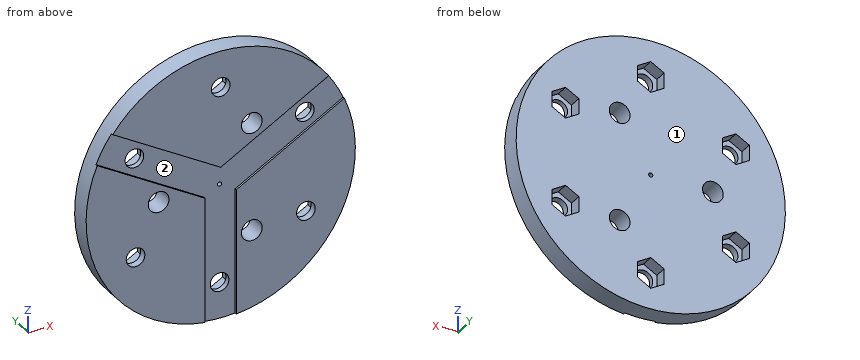
from build123d import *

# Parameters (mm, degrees)
SKETCH1_R           = 65
SKETCH1_R_2         = 1
BOSS_EXTRUDE1_DEPTH = 5
CUT_EXTRUDE1_DEPTH  = 6.4
SKETCH4_R           = 4.5
CUT_EXTRUDE2_DEPTH  = 93.146405247
CUT_EXTRUDE3_START  = -9
CUT_EXTRUDE3_DEPTH  = 3
SKETCH6_R           = 5
CUT_EXTRUDE4_DEPTH  = 93.466210045


with BuildPart() as part:
    # Sketch1 → Boss-Extrude1 (new, symmetric)
    with BuildSketch(Plane(origin=(0, 0, 0), x_dir=(1, 0, 0), z_dir=(0, 1, 0))):
        with Locations(Location((0, 0, 0), (0, 0, 270))):
            Circle(SKETCH1_R)
        with Locations(Location((0, 0, 0), (0, 0, 270))):
            Circle(SKETCH1_R_2, mode=Mode.SUBTRACT)
    extrude(amount=BOSS_EXTRUDE1_DEPTH, both=True)

    # Sketch3 → Cut-Extrude1 (cut)
    with BuildSketch(Plane(origin=(0, 5, 0), x_dir=(1, 0, 0), z_dir=(0, 1, 0))):
        Polygon((34.68620668, 20.026090764), (41.13620668, 16.302181527), (47.58620668, 20.026090764), (47.58620668, 27.473909236), (41.13620668, 31.197818473), (34.68620668, 27.473909236), align=None)
        Polygon((0, 40.052181527), (6.45, 43.776090764), (6.45, 51.223909236), (0, 54.947818473), (-6.45, 51.223909236), (-6.45, 43.776090764), align=None)
        Polygon((34.68620668, -20.026090764), (34.68620668, -27.473909236), (41.13620668, -31.197818473), (47.58620668, -27.473909236), (47.58620668, -20.026090764), (41.13620668, -16.302181527), align=None)
        Polygon((0, -40.052181527), (-6.45, -43.776090764), (-6.45, -51.223909236), (0, -54.947818473), (6.45, -51.223909236), (6.45, -43.776090764), align=None)
        Polygon((-34.68620668, -20.026090764), (-41.13620668, -16.302181527), (-47.58620668, -20.026090764), (-47.58620668, -27.473909236), (-41.13620668, -31.197818473), (-34.68620668, -27.473909236), align=None)
        Polygon((-34.68620668, 20.026090764), (-34.68620668, 27.473909236), (-41.13620668, 31.197818473), (-47.58620668, 27.473909236), (-47.58620668, 20.026090764), (-41.13620668, 16.302181527), align=None)
    extrude(amount=-CUT_EXTRUDE1_DEPTH, mode=Mode.SUBTRACT)

    # Sketch4 → Cut-Extrude2 (cut, through all)
    with BuildSketch(Plane(origin=(0, -1.4, 0), x_dir=(1, 0, 0), z_dir=(0, 1, 0))):
        with Locations(Location((0, 47.5, 0), (0, 0, 270))):
            Circle(SKETCH4_R)
        with Locations(Location((41.13620668, 23.75, 0), (0, 0, 270))):
            Circle(SKETCH4_R)
        with Locations(Location((41.13620668, -23.75, 0), (0, 0, 270))):
            Circle(SKETCH4_R)
        with Locations(Location((0, -47.5, 0), (0, 0, 270))):
            Circle(SKETCH4_R)
        with Locations(Location((-41.13620668, -23.75, 0), (0, 0, 270))):
            Circle(SKETCH4_R)
        with Locations(Location((-41.13620668, 23.75, 0), (0, 0, 270))):
            Circle(SKETCH4_R)
    extrude(amount=-CUT_EXTRUDE2_DEPTH, mode=Mode.SUBTRACT)

    # Sketch5 → Cut-Extrude3 (cut)
    with BuildSketch(Plane(origin=(0, 5, 0), x_dir=(1, 0, 0), z_dir=(0, 1, 0)).offset(CUT_EXTRUDE3_START)):
        Polygon((60.463542815, -26.248388682), (7.5, 4.330127019), (7.5, 65.487158421), (-7.5, 65.487158421), (-7.5, 4.330127019), (-60.463542815, -26.248388682), (-52.963542815, -39.238769739), (0, -8.660254038), (52.963542815, -39.238769739), align=None)
    extrude(amount=-CUT_EXTRUDE3_DEPTH, mode=Mode.SUBTRACT)

    # Sketch6 → Cut-Extrude4 (cut, through all)
    with BuildSketch(Plane.XZ.offset(5)):
        with Locations(Location((-30, 0, 0), (0, 0, 270))):
            Circle(SKETCH6_R)
        with Locations(Location((15, 25.980762114, 0), (0, 0, 270))):
            Circle(SKETCH6_R)
        with Locations(Location((15, -25.980762114, 0), (0, 0, 270))):
            Circle(SKETCH6_R)
    extrude(amount=-CUT_EXTRUDE4_DEPTH, mode=Mode.SUBTRACT)


solid = part.part
Model file for the job. Use its own axes, mm. Face numbers are marked on the shaded views. Coordinates: 2 decimals unless noted, no trailing zeros. Write each loop counter-clockwise with the first axis right and the second up, starting at its lowest first coordinate (ties: lowest second). Pieces come first, ordered by that corner, then holes. Notation, with made-up numbers: (-1.5, 35.25) -> (41.5, 35.25) arc R37 cw to (41.5, 71.25) -> close; hole circle Ø2 at (-0.5, 78). An arc over 180 degrees is marked (long way). One line per item, written item: value. Start each with the question number.
1) Probe probe 1 along X at (y, z) = (0.75, 0); probe 2 along Z at (x, y) = (3.5, 0.75); probe 3 along X at (y, z) = (3.25, -17). List the from-to ranges inside material, lowest first.
2) Slice it at C-C on x = -30. Write the cut outline in (y, z).
3) Flat gauge pins, fed straight in: pin 1 Ø2 at (x, y) = (-36, 4) entering from -Z; pin 2 Ø5 at (y, z) = (0.5, 24.5) entering from +X; pin 3 Ø5 at (x, y) = (-13, 1.5) entering from -Z. Where does each tip first touch, or does it go through?
4) Pull direction Z, two halves, no side cores. Call the marked faces 1 and 2: +Z half, -Z half, draft (parallel to the pull), parting line (faces both ways), or undercut.
5) Slice it at B-B on z = 23.75. Count the separate pieces of the cut face and the enclosed holes in it, then the cut area to 3 significant figures.
6) Slice it at A-A on x = 15. Write the cut outline in (y, z).
7) Slice it at D-D on z = -47.5. Write the cut outline in (x, y).
Answers follow:
1. probe 1: -65 to -35, -25 to -1, 1 to 65
1. probe 2: -64.91 to -52.93, -42.07 to 42.07, 52.93 to 64.91
1. probe 3: -62.74 to -42.34, -39.93 to 39.93, 42.34 to 62.74
2. outline: (-5, -57.66) -> (5, -57.66) -> (5, -5) -> (-5, -5) -> close; (-5, 5) -> (5, 5) -> (5, 57.66) -> (-5, 57.66) -> (-5, 25.98) -> (-4, 25.98) -> (-4, 8.66) -> (-5, 8.66) -> close
3. pin 1: z = -54.77
3. pin 2: x = 61.16
3. pin 3: z = -64.15
4. face 1: draft
4. face 2: undercut
5. separate pieces: 4
5. enclosed holes: 0
5. area: 849 mm2
6. outline: (-5, -63.25) -> (5, -63.25) -> (5, -30.98) -> (-5, -30.98) -> close; (-5, -20.98) -> (5, -20.98) -> (5, 20.98) -> (-5, 20.98) -> (-5, 17.32) -> (-4, 17.32) -> (-4, 0) -> (-5, 0) -> close; (-5, 30.98) -> (5, 30.98) -> (5, 63.25) -> (-5, 63.25) -> close
7. outline: (-44.37, -5) -> (-7.5, -5) -> (-7.5, -4) -> (-4.5, -4) -> (-4.5, -1.4) -> (-6.45, -1.4) -> (-6.45, 5) -> (-44.37, 5) -> close; (4.5, -4) -> (7.5, -4) -> (7.5, -5) -> (44.37, -5) -> (44.37, 5) -> (6.45, 5) -> (6.45, -1.4) -> (4.5, -1.4) -> close
